from build123d import *

# Parameters (mm, degrees)
SKETCH2_W           = 8
SKETCH2_H           = 20
SKETCH2_R           = 2
BOSS_EXTRUDE2_DEPTH = 4
SKETCH3_R           = 2
BOSS_EXTRUDE3_DEPTH = 16
SKETCH5_R           = 2.25
CUT_EXTRUDE1_DEPTH  = 10
CUT_EXTRUDE2_START  = -2
SKETCH6_R           = 4.5
CUT_EXTRUDE2_DEPTH  = 2
SKETCH7_R           = 3.6
CUT_EXTRUDE3_DEPTH  = 16.337861816
SKETCH8_R           = 2
CUT_EXTRUDE4_DEPTH  = 18.066048339


with BuildPart() as part:
    # Sketch2 → Boss-Extrude2 (new body)
    with BuildSketch(Plane(origin=(0, 0, 0), x_dir=(1, 0, 0), z_dir=(0, 1, 0))):
        Rectangle(SKETCH2_W, SKETCH2_H)
        with Locations(Location((0, 6, 0), (0, 0, 270))):
            Circle(SKETCH2_R, mode=Mode.SUBTRACT)
        with Locations(Location((0, -6, 0), (0, 0, 270))):
            Circle(SKETCH2_R, mode=Mode.SUBTRACT)
    extrude(amount=-BOSS_EXTRUDE2_DEPTH)

    # Sketch3 → Boss-Extrude3 (add)
    # profile 1 of 2: a face of its own
    with BuildSketch(Plane.XY.offset(-10)):
        with BuildLine():
            Line((6, 0), (4, 0))
            Line((4, 0), (4, -0.468871126))
            ThreePointArc((4, -0.468871126), (7.027112473, -8.88121444), (6, 0))
        make_face()
        with Locations((6, -4.5)):
            Circle(SKETCH3_R, mode=Mode.SUBTRACT)
    # profile 2 of 2: a face of its own
    with BuildSketch(Plane.XY.offset(-10)):
        with BuildLine():
            Line((-6, 0), (-4, 0))
            Line((-4, 0), (-4, -0.468871126))
            ThreePointArc((-4, -0.468871126), (-7.027112473, -8.88121444), (-6, 0))
        make_face()
        with Locations((-6, -4.5)):
            Circle(SKETCH3_R, mode=Mode.SUBTRACT)
    extrude(amount=BOSS_EXTRUDE3_DEPTH)

    # Sketch5 → Cut-Extrude1 (cut)
    with BuildSketch(Plane.XY.offset(6)):
        with Locations(Location((-6, -4.5, 0), (0, 0, 12.839588407))):
            Circle(SKETCH5_R)
        with Locations(Location((6, -4.5, 0), (0, 0, 152.733955549))):
            Circle(SKETCH5_R)
    extrude(amount=-CUT_EXTRUDE1_DEPTH, mode=Mode.SUBTRACT)

    # Sketch6 → Cut-Extrude2 (cut)
    with BuildSketch(Plane.XY.offset(-4).offset(CUT_EXTRUDE2_START)):
        with Locations((6, -4.5)):
            Circle(SKETCH6_R)
        with Locations((-6, -4.5)):
            Circle(SKETCH6_R)
    extrude(amount=CUT_EXTRUDE2_DEPTH, mode=Mode.SUBTRACT)

    # Sketch7 → Cut-Extrude3 (cut, through all)
    with BuildSketch(Plane.XZ.offset(4)):
        with Locations((0, 6)):
            Circle(SKETCH7_R)
        with Locations((0, -6)):
            Circle(SKETCH7_R)
    extrude(amount=CUT_EXTRUDE3_DEPTH, mode=Mode.SUBTRACT)

    # Sketch8 → Cut-Extrude4 (cut, through all)
    with BuildSketch(Plane(origin=(0, 0, 0), x_dir=(1, 0, 0), z_dir=(0, 1, 0))):
        with Locations(Location((0, 6, 0), (0, 0, 270))):
            Circle(SKETCH8_R)
        with Locations(Location((0, -6, 0), (0, 0, 270))):
            Circle(SKETCH8_R)
    extrude(amount=-CUT_EXTRUDE4_DEPTH, mode=Mode.SUBTRACT)


solid = part.part
Read the model definition and answer for the solid it produces. Units are mm, in the model's axes. A direction names the side the tool comes from. Coordinates: 2 decimals unless noted, no trailing zeros. Write each loop counter-clockwise with the first axis right and the second up, starting at its lowest first coordinate (ties: lowest second). Pieces come first, ordered by that corner, then holes. Notation, with made-up numbers: M -8.75,46.25 L 17.25,46.25 A31 ccw 17.25,74.25 Z; hole C 22,49.5 d10. An arc over 180 degrees is marked long. Use a Markdown table: item, result.
Q1. The part is cut by section A-A, the plane z = 4.75. Write down the section's boundary in (x, y), then the cut area to 3 significant figures.
Answer block:
| item | result |
|---|---|
| outline | M -6,0 A4.5 ccw long -3.38,-8.16 L -3.38,-4 L -1.56,-4 L -1.56,0 Z; M 1.56,-4 L 3.38,-4 L 3.38,-8.16 A4.5 ccw long 6,0 L 1.56,0 Z; hole C -6,-4.5 d4.5; hole C 6,-4.5 d4.5 |
| area | 92.1 mm2 |
Q2. Which of the six approach directions +Z, -Z, +X, -X, +Y, -Y give full straight-line access (tool end or side, diameter ignored) to faces 5 (the face through (8, -3, -6)), 6 (the face through (-8.2, -4.4, -6)), 7 (the face through (-3.264, -6.123, -7.52)), 8 (the face through (0, 0, 0))?
Answer block:
| item | result |
|---|---|
| face 5 | +X, -Y |
| face 6 | -X, -Y |
| face 7 | -Y |
| face 8 | +Z, -Z, +X, -X, +Y |
Q3. The part is cut by section B-B, the plane x = 0. Write down the section's boundary in (y, z), then the cut area to 3 significant figures.
Answer block:
| item | result |
|---|---|
| outline | M -4,-10 L 0,-10 L 0,-8 L -4,-8 Z; M -4,-4 L 0,-4 L 0,4 L -4,4 Z; M -4,8 L 0,8 L 0,10 L -4,10 Z |
| area | 48.0 mm2 |
Q4. Straight lines are drawn through the part: L1, parallel to Z at x = 0, y = -2.05; L2, parallel to X at y = -4.5, z = -0.25; L3, parallel to Y at x = 6, z = -8.75. For each, find the intervals that lie inside material, in ascending order. Write a range as [from, to].
Answer block:
| item | result |
|---|---|
| L1 | z = [-10, -8], [-4, 4], [8, 10] |
| L2 | x = [-10.5, -8.25], [-3.75, -1.5], [1.5, 3.75], [8.25, 10.5] |
| L3 | y = [-9, -6.5], [-2.5, 0] |
Q5. The part is cut by section C-C, the plane y = -7.5. Write down the section's boundary in (x, z), then the cut area to 3 significant figures.
Answer block:
| item | result |
|---|---|
| outline | M -9.35,-10 L -2.65,-10 L -2.65,-8.44 A3.6 cw -3.6,-6 L -9.35,-6 Z; M -9.35,-4 L -2.99,-4 A3.6 cw -2.65,-3.56 L -2.65,3.56 A3.6 cw -3.6,6 L -9.35,6 Z; M 2.65,-10 L 9.35,-10 L 9.35,-6 L 3.6,-6 A3.6 cw 2.65,-8.44 Z; M 2.65,-3.56 A3.6 cw 2.99,-4 L 9.35,-4 L 9.35,6 L 3.6,6 A3.6 cw 2.65,3.56 Z |
| area | 181 mm2 |
Q6. The part is cut by section D-D, the plane z = -8.25. Write down the section's boundary in (x, y).
Answer block:
| item | result |
|---|---|
| outline | M -6,0 A4.5 ccw long -2.81,-7.67 L -2.81,-4 L 2.81,-4 L 2.81,-7.67 A4.5 ccw long 6,0 Z; hole C -6,-4.5 d4; hole C 6,-4.5 d4 |
Q7. Determine the mould class of faces 1 (the face through (-4, -2, 8)), 2 (the face through (-8.89, -7.95, 0.93)), 3 (the face through (7, -2, -4)), 4 (the face through (3.62, -0.68, -5.01)) for opening direction X: released by +X, released by -X, zero draft, split by the parting line, or undercut.
Answer block:
| item | result |
|---|---|
| face 1 | released by -X |
| face 2 | undercut |
| face 3 | zero draft |
| face 4 | released by +X |
Q8. Each of these flat-tipped pins is pushed along its axis until it touches: pin 1 Ø4 at (y, z) = (-7, -2) entering from +X; pin 2 Ø5 at (x, z) = (0, 6) entering from -Y; pin 3 Ø2.5 at (x, z) = (-1, 1) entering from -Y; pin 4 Ø4 at (y, z) = (-4, 7) entering from -X. Where does it stop, or does it pass through?
Answer block:
| item | result |
|---|---|
| pin 1 | stops at x = 10.47 |
| pin 2 | stops at y = -4 |
| pin 3 | stops at y = -6.99 |
| pin 4 | stops at x = -10.5 |
